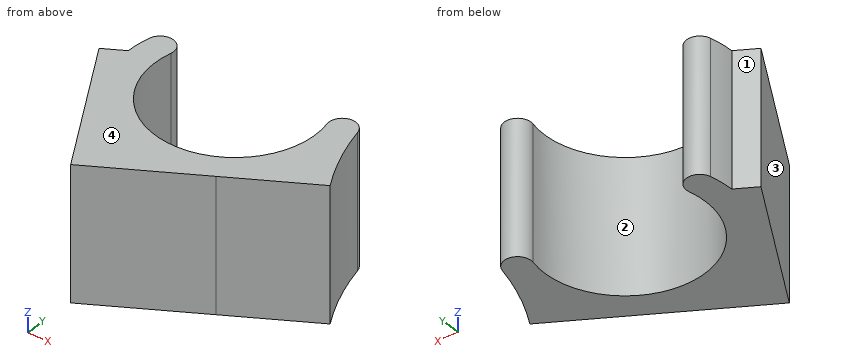
Autodesk Inventor part; units mm, degrees
ref_plane "YZ Plane" through (0, 0, 0) normal (1, 0, 0) x (0, 1, 0)
ref_plane "XZ Plane" through (0, 0, 0) normal (0, 1, 0) x (-1, 0, 0)
ref_plane "XY Plane" through (0, 0, 0) normal (0, 0, 1) x (1, 0, 0)
sketch "Skizze1" plane through (0, 0, 0) normal (0, 0, 1) x (1, 0, 0)
  circle A0 centre (0, 0) radius 9
  circle A1 centre (0, 0) radius 12
  arc A2 (-8.775, 2) -> (-11.7, 2.6667) centre (-10.2375, 2.3333) ccw
  arc A3 (11.7, 2.6667) -> (8.775, 2) centre (10.2375, 2.3333) ccw
  line L0 (-12, 0) -> (-14.2583, -1.3038)
  line L1 (-14.2583, -1.3038) -> (-5.2583, -16.8923)
  line L2 (-5.2583, -16.8923) -> (6, -10.3923)
  line L3 (0, -22.6708) -> (0, 17.7785)
  line L4 (6, -10.3923) -> (14.8243, -5.2976)
  arc A4 (11.7, 2.6667) -> (14.8243, -5.2976) centre (39.6544, 9.0381) ccw
  dimension "d0" = 18
  dimension "d1" = 3
  dimension "d2" = 2
  dimension "d4" = 18
  dimension "d5" = 13
  dimension "d6" = 120
extrude "Extrusion1" add sketch "Skizze1" along normal mid plane 15 contours A0 A3 A1 L3 | L3 A1 A2 A0 | A4 L4 A1 | L3 L2 L1 L0 A1 | A1 L2 L3 picked at (10.9126, -0.8316) picked at (-1.5575, -10.8245)
properties part number "baztholder_3D-Druck"
Work out the finished part from the listing and answer in its coordinate system (mm). Face numbers are marked on the shaded views. Give positions to 0.01 mm unless a question says otherwise; leave off trailing zeros. Loops run counter-clockwise (first coordinate to the right, second up) from the corner with the lowest first, then second, coordinate; pieces in that order, holes last. Notation, with made-up numbers: (-24.5, 68.25) - (-13.5, 68.25) arc R20 cw to (-13.5, 104.25) - close; hole circle Ø8 at (-20.5, 66). An arc over 180 degrees is marked (long way). One line per question, with ' | ' between items.
(1) The part is cut by section B-B (z = 0). Write down the section's boundary in (x, y) (1 decimal).
Recorded:
outline: (-14.3, -1.3) - (-5.3, -16.9) - (6, -10.4) - (14.8, -5.3) arc R28.7 cw to (11.7, 2.7) arc R1.5 ccw to (8.8, 2) arc R9 cw (long way) to (-8.8, 2) arc R1.5 ccw to (-11.7, 2.7) arc R12 ccw to (-12, 0) - close
(2) Each of these flat-tipped pins is pushed along its axis until it touches: pin 1 Ø6 at (y, z) = (-1, 0) entering from +X; pin 2 Ø8 at (y, z) = (-8.5, -1) entering from +X; pin 3 Ø6 at (x, z) = (0, 5) entering from -Y; pin 4 Ø12 at (x, y) = (-6.5, -3.5) entering from -Z. Where does it stop, or does it pass through?
Recorded:
pin 1: stops at x = 14.12 | pin 2: stops at x = 14.82 | pin 3: stops at y = -15.59 | pin 4: stops at z = -7.5
(3) The part is cut by section C-C (x = 0). Write down the section's boundary in (y, z).
Recorded:
outline: (-13.86, -7.5) - (-9, -7.5) - (-9, 7.5) - (-13.86, 7.5) - close
(4) Straight lines are drawn through the part: probe 1 along X at (y, z) = (2.75, -5.75); probe 2 along X at (y, z) = (1, 6.5); probe 3 along Y at (x, z) = (0.5, 3). For each, find the intervals that lie inside material, in ascending order.
Recorded:
probe 1: x = -11.68 to -8.8, 8.8 to 11.68 | probe 2: x = -11.96 to -8.94, 8.94 to 12.13 | probe 3: y = -13.57 to -8.99
(5) The mould has two halves that part along Y. Classify the marked faces 1, 2, 3 and 4: +Y half, -Y half, draft (parallel to the pull), parting line (faces both ways), or undercut.
Recorded:
face 1: +Y half | face 2: undercut | face 3: -Y half | face 4: draft
(6) The part is cut by section D-D (y = -13.25). Write down the section's boundary in (x, z), then the cut area to 3 significant figures.
Recorded:
outline: (-7.36, -7.5) - (1.05, -7.5) - (1.05, 7.5) - (-7.36, 7.5) - close | area: 126 mm²
(7) The part is cut by section A-A (y = -7.25). Write down the section's boundary in (x, z), then the cut area to 3 significant figures.
Recorded:
outline: (-10.83, -7.5) - (-5.33, -7.5) - (-5.33, 7.5) - (-10.83, 7.5) - close; (5.33, -7.5) - (11.44, -7.5) - (11.44, 7.5) - (5.33, 7.5) - close | area: 174 mm²
